Build history of the part. All positions in model axes, mm. Face numbers are marked on the shaded views. A direction names the side the tool comes from. Round coordinates to 2 decimals unless told otherwise and drop trailing zeros. One line per question, with ' | ' between items. Start each with the question number.
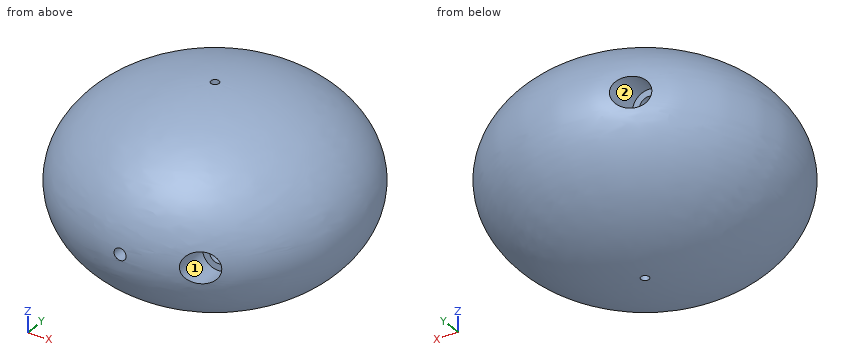
from build123d import *

# Parameters (mm, degrees)
CUT_EXTRUDE2_DEPTH      = 42.041138069
CUT_EXTRUDE2_DEPTH_BACK = 42.041138069
SKETCH4_R               = 0.75
CUT_EXTRUDE3_START      = -27
CUT_EXTRUDE3_OUTLINE_R  = 1.1
CUT_EXTRUDE3_DEPTH      = 27.0001
SKETCH6_R               = 2.05
CUT_EXTRUDE4_DEPTH      = 10
SKETCH6_5_R             = 2.05
CUT_EXTRUDE10_DEPTH     = 10
CUT_EXTRUDE8_REACH      = 43.038
SKETCH6_4_R             = 1.6
CUT_EXTRUDE11_REACH     = 43.038
SKETCH6_6_R             = 1.6
CUT_EXTRUDE9_REACH      = 61.038
CUT_EXTRUDE9_START      = -18
SKETCH11_R              = 2.85
CUT_EXTRUDE12_REACH     = 61.038
CUT_EXTRUDE12_START     = 18
SKETCH11_3_R            = 2.85
SKETCH12_R              = 2.05
CUT_EXTRUDE13_DEPTH     = 8
CHAMFER1_SIZE           = 1.5


with BuildPart() as part:
    # Sketch1 → Revolve4 (revolve)
    with BuildSketch(Plane(origin=(0, 0, 0), x_dir=(1, 0, 0), z_dir=(0, 1, 0))):
        with BuildLine():
            Line((0, 17.5), (0, -17.5))
            add(Edge.make_bspline(
                [(0, -17.5), (26.25, -17.5), (26.25, 0), (26.25, 17.5), (0, 17.5)],
                knots=[1.570796327, 1.570796327, 1.570796327, 3.141592654, 3.141592654, 4.71238898, 4.71238898, 4.71238898], degree=2, weights=[1, 0.707106781, 1, 0.707106781, 1]))
        make_face()
    revolve(axis=Axis((0, 0, -17.5), (0, 0, 1)))

    # Sketch4 → Cut-Extrude2 (cut, two sides: drawn at the far end of the back side and taken through both)
    with BuildSketch(Plane.XY.offset(-CUT_EXTRUDE2_DEPTH_BACK)):
        with Locations(Location((0, 0, 0), (0, 0, 180))):
            Circle(SKETCH4_R)
    extrude(amount=CUT_EXTRUDE2_DEPTH + CUT_EXTRUDE2_DEPTH_BACK, mode=Mode.SUBTRACT)

    # Cut-Extrude3: read off the stored shape, not the designer's step
    # Cut-Extrude3 outline → Cut-Extrude3 (cut)
    with BuildSketch(Plane(origin=(0, 0, 0), x_dir=(1, 0, 0), z_dir=(0, 1, 0)).offset(CUT_EXTRUDE3_START)):
        Circle(CUT_EXTRUDE3_OUTLINE_R)
    extrude(amount=CUT_EXTRUDE3_DEPTH, mode=Mode.SUBTRACT)

    # Sketch6 → Cut-Extrude4 (cut)
    with BuildSketch(Plane(origin=(0, 0, 0), x_dir=(1, 0, 0), z_dir=(0, 1, 0))):
        with Locations(Location((-12.5, 0, 0), (0, 0, 270))):
            Circle(SKETCH6_R)
    extrude(amount=-CUT_EXTRUDE4_DEPTH, mode=Mode.SUBTRACT)

    # Sketch6<5> → Cut-Extrude10 (cut)
    with BuildSketch(Plane(origin=(0, 0, 0), x_dir=(1, 0, 0), z_dir=(0, 1, 0))):
        with Locations(Location((12.5, 0, 0), (0, 0, 270))):
            Circle(SKETCH6_5_R)
    extrude(amount=CUT_EXTRUDE10_DEPTH, mode=Mode.SUBTRACT)

    # Sketch6<4> → Cut-Extrude8 (cut, up to next)
    with BuildSketch(Plane(origin=(0, 0, 0), x_dir=(1, 0, 0), z_dir=(0, 1, 0)), mode=Mode.PRIVATE) as cut_extrude8_sk1:
        with Locations(Location((12.5, 0, 0), (0, 0, 270))):
            Circle(SKETCH6_4_R)
    cut_extrude8_tool1 = extrude(cut_extrude8_sk1.sketch, amount=-CUT_EXTRUDE8_REACH, mode=Mode.PRIVATE) & part.part
    add(cut_extrude8_tool1.solids().sort_by_distance((12.5, 0, 0))[0], mode=Mode.SUBTRACT)

    # Sketch6<6> → Cut-Extrude11 (cut, up to next)
    with BuildSketch(Plane(origin=(0, 0, 0), x_dir=(1, 0, 0), z_dir=(0, 1, 0)), mode=Mode.PRIVATE) as cut_extrude11_sk1:
        with Locations(Location((-12.5, 0, 0), (0, 0, 90))):
            Circle(SKETCH6_6_R)
    cut_extrude11_tool1 = extrude(cut_extrude11_sk1.sketch, amount=CUT_EXTRUDE11_REACH, mode=Mode.PRIVATE) & part.part
    add(cut_extrude11_tool1.solids().sort_by_distance((-12.5, 0, 0))[0], mode=Mode.SUBTRACT)

    # Sketch11 → Cut-Extrude9 (cut, up to next)
    with BuildSketch(Plane(origin=(0, 0, 0), x_dir=(1, 0, 0), z_dir=(0, 1, 0)).offset(CUT_EXTRUDE9_START), mode=Mode.PRIVATE) as cut_extrude9_sk1:
        with Locations(Location((12.5, 0, 0), (0, 0, 270))):
            Circle(SKETCH11_R)
    cut_extrude9_tool1 = extrude(cut_extrude9_sk1.sketch, amount=-CUT_EXTRUDE9_REACH, mode=Mode.PRIVATE) & part.part
    add(cut_extrude9_tool1.solids().sort_by_distance((12.5, -18, 0))[0], mode=Mode.SUBTRACT)

    # Sketch11<3> → Cut-Extrude12 (cut, up to next)
    with BuildSketch(Plane(origin=(0, 0, 0), x_dir=(1, 0, 0), z_dir=(0, 1, 0)).offset(CUT_EXTRUDE12_START), mode=Mode.PRIVATE) as cut_extrude12_sk1:
        with Locations(Location((-12.5, 0, 0), (0, 0, 90))):
            Circle(SKETCH11_3_R)
    cut_extrude12_tool1 = extrude(cut_extrude12_sk1.sketch, amount=CUT_EXTRUDE12_REACH, mode=Mode.PRIVATE) & part.part
    add(cut_extrude12_tool1.solids().sort_by_distance((-12.5, 18, 0))[0], mode=Mode.SUBTRACT)

    # Sketch12 → Cut-Extrude13 (cut)
    with BuildSketch(Plane(origin=(0, 0, 0), x_dir=(1, 0, 0), z_dir=(0, 1, 0))):
        with Locations(Location((0, 0, 0), (0, 0, 270))):
            Circle(SKETCH12_R)
    extrude(amount=-CUT_EXTRUDE13_DEPTH, mode=Mode.SUBTRACT)

    # Chamfer1
    # the kernel refuses this chamfer: 1.5 mm, written as the material it adds along each edge
    with BuildSketch(Plane(origin=(0, -8, 0), x_dir=(0, 0, 1), z_dir=(-1, 0, 0))) as chamfer1_piece_1_section:
        Polygon((2.05 - CHAMFER1_SIZE, 0), (2.05, CHAMFER1_SIZE), (2.05, 0), align=None)
    chamfer1_piece_1 = revolve(axis=Axis((0, -8, 0), (0, 1, 0)), mode=Mode.PRIVATE)
    chamfer1_piece_1 = chamfer1_piece_1 - Plane(origin=(0, -8, 0), x_dir=(1, 0, 0), z_dir=(0, -1, 0)) * Cylinder(1.1, 9, mode=Mode.PRIVATE)
    add(chamfer1_piece_1)


solid = part.part
Item 1: Flat gauge pins, fed straight in: pin 1 (6.5 mm diameter, centred on x = 12.5, z = 0, fed in from -Y); pin 2 (2 mm diameter, centred on x = 18, y = -13.5, fed in from -Z); pin 3 (2 mm diameter, centred on x = 6.5, y = 0, fed in from +Z); pin 4 (2.5 mm diameter, centred on x = 0, z = 0, fed in from -Y). Where does each tip first touch, or does it go through?
Item 2: Cut at A-A on y = -4.5. Count the separate pieces of the cut face and the enclosed holes in it, then the cut area to 3 significant figures.
Item 3: Tool access for the marked faces 1 and 2: list every direction of +Z, -Z, +X, -X, +Y, -Y with a clear straight run to the whole face (end or side of a thin tool).
Item 4: Wall check: line 1 along X through (y, z) = (3, -1); line 2 along X through (y, z) = (-4.75, 0); line 3 along Z through (x, y) = (0, -1). Give the ranges that are in metal, low to high. Write a range as [from, to].
Results found:
1) pin 1: stops at y = -24.57 | pin 2: stops at z = -10.04 | pin 3: stops at z = 17.11 | pin 4: stops at y = -26.23
2) separate pieces: 1 | enclosed holes: 3 | area: 1,370 mm^2
3) face 1: -Y | face 2: +Y
4) line 1: x = [-26.03, -13.75], [-11.25, 10.71], [14.29, 26.03] | line 2: x = [-25.82, -14.55], [-10.45, -2.05], [2.05, 10.9], [14.1, 25.82] | line 3: z = [-17.49, -2.05], [2.05, 17.49]
